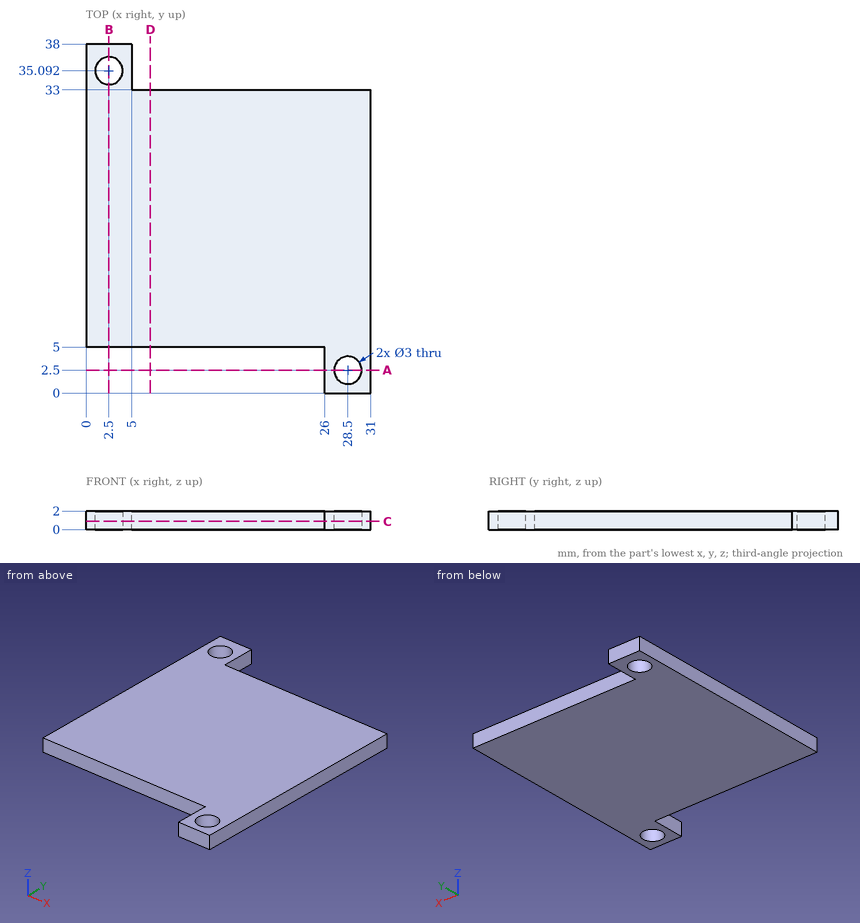
Drawing for the job (mm, zero at the part's lowest x, y, z). Round coordinates to 2 decimals unless told otherwise and drop trailing zeros. Order: outer loops, then holes, each group sorted by start corner. A loop starts at its lowest first (then second) coordinate and runs counter-clockwise, first axis right, second up. Notation, with made-up numbers: M 30,-11 L 59,-11 A17 cw 59,7 Z; hole C 9,24 d9. An arc over 180 degrees is marked long. Use one line per item in the form item = value.
Q1. Saw through at D-D on x = 7. Give the cut face in (y, z), then the cut area to 3 significant figures.
Recorded:
outline = M 5,0 L 33,0 L 33,2 L 5,2 Z
area = 56.0 mm^2
Q2. Probe L1, parallel to Y at x = 28.5, z = 0.9; L2, parallel to Y at x = 6, z = 1.6; L3, parallel to Y at x = 2.5, z = 1.45. List the from-to ranges inside material, lowest first.
Recorded:
L1 = 0 to 1, 4 to 33
L2 = 5 to 33
L3 = 5 to 33.59, 36.59 to 38
Q3. Saw through at C-C on z = 0.9. Give the cut face in (x, y), then the cut area to 3 significant figures.
Recorded:
outline = M 0,5 L 26,5 L 26,0 L 31,0 L 31,33 L 5,33 L 5,38 L 0,38 Z; hole C 2.5,35.09 d3; hole C 28.5,2.5 d3
area = 904 mm^2
Q4. Saw through at A-A on y = 2.5. Give the cut face in (x, z), then the cut area to 3 significant figures.
Recorded:
outline = M 26,0 L 27,0 L 27,2 L 26,2 Z; M 30,0 L 31,0 L 31,2 L 30,2 Z
area = 4.00 mm^2
Q5. Saw through at B-B on x = 2.5. Give the cut face in (y, z), then the cut area to 3 significant figures.
Recorded:
outline = M 5,0 L 33.59,0 L 33.59,2 L 5,2 Z; M 36.59,0 L 38,0 L 38,2 L 36.59,2 Z
area = 60.0 mm^2
Q6. Flat gauge pins, fed straight in: P1, Ø1, axis at x = 6.5, z = 1, coming from the -Y side; P2, Ø1, axis at x = 13, z = 0.5, coming from the +Y side; P3, Ø0.6, axis at y = 3.5, z = 1, coming from the -X side. Where does each tip first touch, or does it go through?
Recorded:
P1 = 5
P2 = 33
P3 = 26
